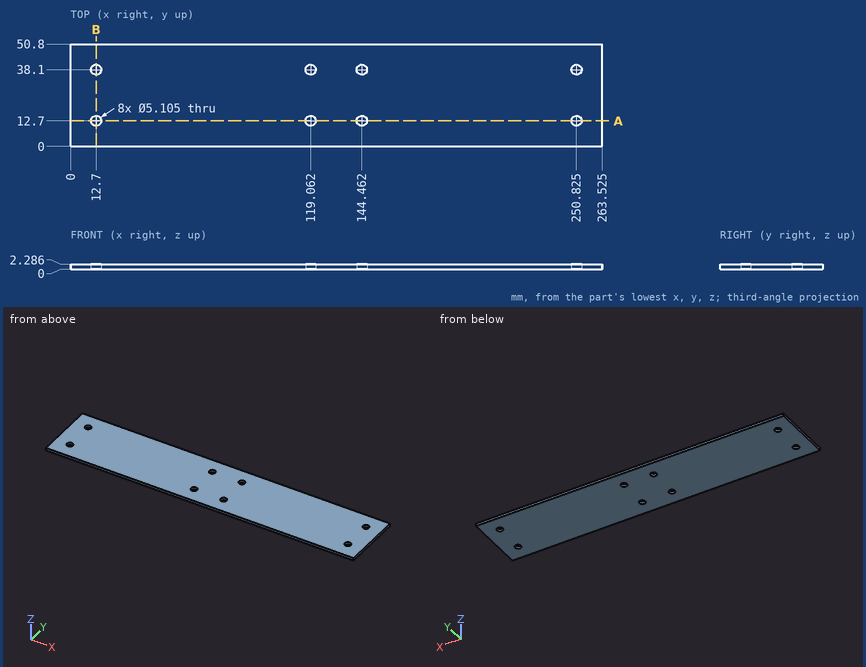
Geometry check sheet. Reference: drawing and pictorial views, mm from the part's lowest x, y, z. Round coordinates to 2 decimals unless told otherwise and drop trailing zeros. Order: outer loops, then holes, each group sorted by start corner. A loop starts at its lowest first (then second) coordinate and runs counter-clockwise, first axis right, second up. Notation, with made-up numbers: (7, 33) -> (53, 33) arc R26 ccw to (53, 67) -> close; hole circle Ø6 at (58, -39). An arc over 180 degrees is marked (long way). One line per item, written item: value. Start each with the question number.
Q1. Cross-section at A-A (y = 12.7). Record the boundary of the cut face in (x, z) (1 decimal).
Q2. Cross-section at B-B (x = 12.7). Record the boundary of the cut face in (y, z) (1 decimal).
Q3. Thickness scan on line 1 (Y direction, x = 250.5, z = 1.4); line 2 (X direction, y = 38.1, z = 1.55) (1 decimal); line 3 (Y direction, x = 12.7, z = 1.4). Record the ranges inside material, lowest first.
Completed:
1. outline: (0, 0) -> (10.1, 0) -> (10.1, 2.3) -> (0, 2.3) -> close; (15.3, 0) -> (116.5, 0) -> (116.5, 2.3) -> (15.3, 2.3) -> close; (121.6, 0) -> (141.9, 0) -> (141.9, 2.3) -> (121.6, 2.3) -> close; (147, 0) -> (248.3, 0) -> (248.3, 2.3) -> (147, 2.3) -> close; (253.4, 0) -> (263.5, 0) -> (263.5, 2.3) -> (253.4, 2.3) -> close
2. outline: (0, 0) -> (10.1, 0) -> (10.1, 2.3) -> (0, 2.3) -> close; (15.3, 0) -> (35.5, 0) -> (35.5, 2.3) -> (15.3, 2.3) -> close; (40.7, 0) -> (50.8, 0) -> (50.8, 2.3) -> (40.7, 2.3) -> close
3. line 1: y = 0 to 10.17, 15.23 to 35.57, 40.63 to 50.8
3. line 2: x = 0 to 10.1, 15.3 to 116.5, 121.6 to 141.9, 147 to 248.3, 253.4 to 263.5
3. line 3: y = 0 to 10.15, 15.25 to 35.55, 40.65 to 50.8
